from build123d import *

# Parameters (mm, degrees)
BOSS_EXTRUDE1_DEPTH = 5
SKETCH2_R           = 2.5
CUT_EXTRUDE1_DEPTH  = 41.620192023
SKETCH3_W           = 5
SKETCH3_H           = 15
BOSS_EXTRUDE2_DEPTH = 2
FILLET1_START       = -35
FILLET1_DEPTH       = 5
FILLET1_START_2     = 30
FILLET1_2_DEPTH     = 5
FILLET1_START_3     = -5
FILLET1_3_DEPTH     = 10
FILLET1_4_DEPTH     = 5
FILLET1_5_DEPTH     = 5
FILLET1_6_DEPTH     = 10


with BuildPart() as part:
    # Sketch1 → Boss-Extrude1 (new, symmetric)
    with BuildSketch(Plane(origin=(0, 0, 0), x_dir=(1, 0, 0), z_dir=(0, 1, 0))):
        Polygon((-35, 15), (35, 15), (35, -15), (30, -15), (30, 5), (-30, 5), (-30, -15), (-35, -15), align=None)
    extrude(amount=BOSS_EXTRUDE1_DEPTH, both=True)

    # Sketch2 → Cut-Extrude1 (cut, through all)
    with BuildSketch(Plane.XY.offset(-5)):
        Circle(SKETCH2_R)
    extrude(amount=-CUT_EXTRUDE1_DEPTH, mode=Mode.SUBTRACT)

    # Sketch3 → Boss-Extrude2 (add)
    with BuildSketch(Plane.XY.offset(15)):
        with Locations((-32.5, -2.5)):
            Rectangle(SKETCH3_W, SKETCH3_H)
        with Locations((32.5, 2.5)):
            Rectangle(SKETCH3_W, SKETCH3_H)
    extrude(amount=-BOSS_EXTRUDE2_DEPTH)

    # Fillet1: read off the stored shape, not the designer's step
    # Fillet1 outline → Fillet1 (add)
    with BuildSketch(Plane.YZ.offset(FILLET1_START)):
        with BuildLine():
            Line((-5, 13), (-10, 13))
            ThreePointArc((-10, 13), (-6.464466094, 11.535533906), (-5, 8))
            Line((-5, 8), (-5, 13))
        make_face()
    extrude(amount=FILLET1_DEPTH)

    # Fillet1 2 outline → Fillet1 2 (add)
    with BuildSketch(Plane.YZ.offset(FILLET1_START_2)):
        with BuildLine():
            Line((5, 13), (5, 8))
            ThreePointArc((5, 8), (6.464466094, 11.535533906), (10, 13))
            Line((10, 13), (5, 13))
        make_face()
    extrude(amount=FILLET1_2_DEPTH)

    # Fillet1 3 outline → Fillet1 3 (add)
    with BuildSketch(Plane(origin=(0, 0, 0), x_dir=(1, 0, 0), z_dir=(0, 1, 0)).offset(FILLET1_START_3)):
        with BuildLine():
            Line((-30, 5), (-30, 0))
            ThreePointArc((-30, 0), (-28.535533906, 3.535533906), (-25, 5))
            Line((-25, 5), (-30, 5))
        make_face()
        with BuildLine():
            Line((30, 5), (25, 5))
            ThreePointArc((25, 5), (28.535533906, 3.535533906), (30, 0))
            Line((30, 0), (30, 5))
        make_face()
    extrude(amount=FILLET1_3_DEPTH)

    # Fillet1 4 outline → Fillet1 4 (cut)
    with BuildSketch(Plane.YZ.offset(FILLET1_START)):
        with BuildLine():
            Line((5, 15), (0, 15))
            ThreePointArc((0, 15), (3.535533906, 13.535533906), (5, 10))
            Line((5, 10), (5, 15))
        make_face()
    extrude(amount=FILLET1_4_DEPTH, mode=Mode.SUBTRACT)

    # Fillet1 5 outline → Fillet1 5 (cut)
    with BuildSketch(Plane.YZ.offset(FILLET1_START_2)):
        with BuildLine():
            Line((-5, 15), (-5, 10))
            ThreePointArc((-5, 10), (-3.535533906, 13.535533906), (0, 15))
            Line((0, 15), (-5, 15))
        make_face()
    extrude(amount=FILLET1_5_DEPTH, mode=Mode.SUBTRACT)

    # Fillet1 6 outline → Fillet1 6 (cut)
    with BuildSketch(Plane(origin=(0, 0, 0), x_dir=(1, 0, 0), z_dir=(0, 1, 0)).offset(FILLET1_START_3)):
        with BuildLine():
            Line((-35, 15), (-35, 10))
            ThreePointArc((-35, 10), (-33.535533906, 13.535533906), (-30, 15))
            Line((-30, 15), (-35, 15))
        make_face()
        with BuildLine():
            Line((35, 15), (30, 15))
            ThreePointArc((30, 15), (33.535533906, 13.535533906), (35, 10))
            Line((35, 10), (35, 15))
        make_face()
    extrude(amount=FILLET1_6_DEPTH, mode=Mode.SUBTRACT)


solid = part.part
Check sheet for the modelled part. Datum: model origin and axes. Units: mm. A direction names the side the tool comes from. Give positions to 0.01 mm unless a question says otherwise; leave off trailing zeros. Write each loop counter-clockwise with the first axis right and the second up, starting at its lowest first coordinate (ties: lowest second). Pieces come first, ordered by that corner, then holes. Notation, with made-up numbers: (-29.75, 5) -> (13.25, 5) arc R29 ccw to (13.25, 34) -> close; hole circle Ø10 at (50, 30.25). An arc over 180 degrees is marked (long way). Use one line per item in the form item = value. Start each with the question number.
1. Section check D-D (z = -8). Record the cut outline in (x, y), and give its area (3 significant figures).
2. Thickness scan on line 1 along Y through (x, z) = (0, -9.5); line 2 along X through (y, z) = (-1.25, -2.75); line 3 along Z through (x, y) = (-15, 2). Record the ranges inside material, lowest first. Write a range as from..to.
3. Section check C-C (y = -1.75). Record the cut outline in (x, z), and give its area (3 significant figures).
4. Access from +Z, -Z, +X, -X, +Y, -Y to the whole of each face (thin tool, end or side, straight path). Record for faces 5 (the cylindrical face through (-33, -7, 12)), 6 (the flat face through (0, 3, -5)), 7 (the cylindrical face through (32, -4, 13)).
5. Section check B-B (z = -3.25). Record the cut outline in (x, y).
6. Go/stop test with flat-tipped pins: P1, Ø8, axis at x = 13.5, z = -6, coming from the -Y side; P2, Ø3, axis at x = 11, y = 0, coming from the +Z side; P3, Ø3, axis at x = -23, z = -9, coming from the +Y side. Record where each tip stops, or that it passes through.
7. Section check A-A (x = 0). Record the cut outline in (y, z).
8. Mould release check, pull along X, two halves, no side actions. Record for faces 1 (the flat face through (-33, -5, 15)), 2 (the cylindrical face through (33, 0, -14)), 3 (the cylindrical face through (28, 0, -4)), 4 (the flat face through (-30, -1, 8)): pulls with the +X half, pulls with the -X half, needs draft (parallel to the pull), parting line crosses it, or undercut.
Conclusion:
q1.outline = (-35, -5) -> (35, -5) -> (35, 5) -> (-35, 5) -> close; hole circle Ø5 at (0, 0)
q1.area = 680 mm²
q2.line_1 = -5..-2.5, 2.5..5
q2.line_2 = -35..-29.18, 29.18..35
q2.line_3 = -15..-5
q3.outline = (-35, -10) arc R5 ccw to (-30, -15) -> (-1.79, -15) -> (-1.79, -5) -> (-25, -5) arc R5 cw to (-30, 0) -> (-30, 15) -> (-35, 15) -> close; (1.79, -15) -> (30, -15) arc R5 ccw to (35, -10) -> (35, 14.68) -> (30, 14.68) -> (30, 0) arc R5 cw to (25, -5) -> (1.79, -5) -> close
q3.area = 863 mm²
q4.face_5 = -Z, +X, -X, -Y
q4.face_6 = +Z, +Y, -Y
q4.face_7 = +Z, +X, -Y
q5.outline = (-35, -5) -> (-28.8, -5) -> (-28.8, 5) -> (-35, 5) -> close; (28.8, -5) -> (35, -5) -> (35, 5) -> (28.8, 5) -> close
q6.P1 = -5
q6.P2 = -5
q6.P3 = 5
q7.outline = (-5, -15) -> (-2.5, -15) -> (-2.5, -5) -> (-5, -5) -> close; (2.5, -15) -> (5, -15) -> (5, -5) -> (2.5, -5) -> close
q8.face_1 = needs draft
q8.face_2 = pulls with the +X half
q8.face_3 = undercut
q8.face_4 = undercut
